The listing builds one solid part. Answer for the finished solid, in the listing's coordinates (mm). Face numbers are marked on the shaded views. A direction names the side the tool comes from. Round coordinates to 2 decimals unless told otherwise and drop trailing zeros. Write each loop counter-clockwise with the first axis right and the second up, starting at its lowest first coordinate (ties: lowest second). Pieces come first, ordered by that corner, then holes. Notation, with made-up numbers: M 47,-30 L 61,-30 A15 cw 61,-19 Z; hole C 61,48.5 d6. An arc over 180 degrees is marked long. One line per item, written item: value. Start each with the question number.
(1) Consider probe 1 along Z at (x, y) = (0, 2.5); probe 2 along Y at (x, z) = (3.5, 3). Determine where each line is inside the solid, lowest interval first.
(2) Section C-C (y = 1.6) is taken. Determine the outline of the cut face in (x, z) (1 decimal).
(3) For the marked faces 1 and 2, determine the directions among +Z, -Z, +X, -X, +Y, -Y from which every point of the face is accessible in a straight line to the end or side of a thin tool.
(4) Given P1, Ø1, axis at y = 3, z = 0.5, coming from the +X side; P2, Ø2, axis at y = 3, z = -3, coming from the -X side, each flat-ended and moving along its own axis, determine where each tip first touches the part or whether it passes through.
```python
from build123d import *

# Parameters (mm, degrees)
FILLET1_R = 0.5


with BuildPart() as part:
    # Sketch1 → Revolve1 (revolve)
    with BuildSketch(Plane(origin=(0, 0, 0), x_dir=(0, 0, -1), z_dir=(1, 0, 0))):
        Polygon((0, 0), (0, 4), (-4.5125, 4), (-4.5125, 1), (-5.5125, 1), (-5.5125, 0), align=None)
    revolve(axis=Axis((0, 0, 0), (0, -1, 0)))

    # Fillet1
    fillet1_edges = [part.edges().sort_by_distance(p)[0] for p in [
        (0, 0, -5.5125),
        (0, 1, -5.5125),
        (0, 4, -4.5125),
    ]]
    fillet(fillet1_edges, radius=FILLET1_R - 0.0001)  # a hair under: the kernel refuses the full size


solid = part.part
```
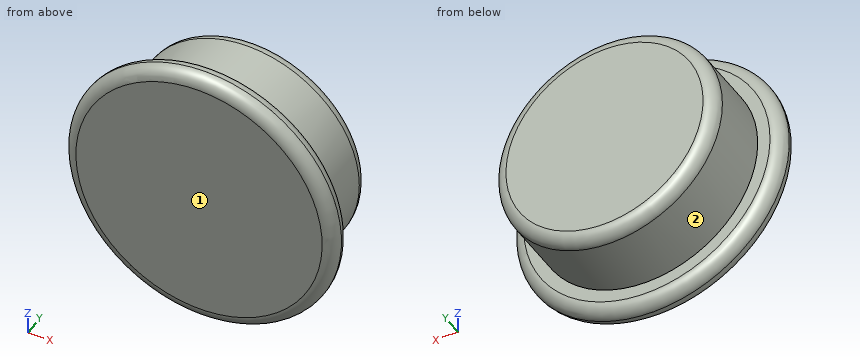
Recorded:
1. probe 1: z = -4.51 to 4.51
1. probe 2: y = 0 to 1
2. outline: C 0,0 d9
3. face 1: +Z, -Z, +X, -X, -Y
3. face 2: +Y
4. P1: stops at x = 4.51
4. P2: stops at x = -4.05
